Could you check a few things on this model? Use its own coordinates, in mm. Give positions to 0.01 mm unless a question says otherwise; leave off trailing zeros. Loops run counter-clockwise (first coordinate to the right, second up) from the corner with the lowest first, then second, coordinate; pieces in that order, holes last. Notation, with made-up numbers: M -21.5,7 L -1.5,7 A18 cw -1.5,11 Z; hole C 83,32 d9. An arc over 180 degrees is marked long. Write each question's results on one line, items separated by ' | '. Start each with the question number.
from build123d import *

# Parameters (mm, degrees)
F0_R     = 3.175
F1_DEPTH = 31.75
F3_D     = 3.175
F3_DEPTH = 12.7
F3_TIP   = 0.9538662327
F4_SIZE2 = 0.8798818102
F4_SIZE  = 1.524


with BuildPart() as f1:
    # F0 (on Front) → F1 (new body)
    with BuildSketch(Plane.XZ):
        Circle(F0_R)
    extrude(amount=F1_DEPTH)

    # F3
    with Locations(Plane.XZ.offset(31.75)):
        with Locations((0, 0)):
            Hole(F3_D / 2, depth=F3_DEPTH)
            with Locations((0, 0, -(F3_DEPTH + F3_TIP / 2))):  # 118° drill point
                Cone(0, F3_D / 2, F3_TIP, mode=Mode.SUBTRACT)

    # F4
    f4_edges = [f1.edges().sort_by_distance(p)[0] for p in [
        (-3.175, 0, 0),
    ]]
    f4_side = f1.faces().sort_by_distance((-3.175, -15.875, 0))[0]
    chamfer(f4_edges, length=F4_SIZE, length2=F4_SIZE2, reference=f4_side)


solid = f1.part
1) I'm going to push a flat-ended pin straight in: P1, Ø3, axis at x = 0, z = 0, coming from the -Y side. Where does the tip first touch, or does it pass through?
2) Please list where these lines run through material, in increasing order: line 1 (Z direction, x = 0, y = -24) (1 decimal); line 2 (Z direction, x = -0.5, y = -20); line 3 (X direction, y = -26.5, z = 0.75). Write a range as from..to.
3) Thinking about a two-plate mould opening in Z: for faces 1 (the face through (1.4, -31.75, -1.4)), 2 (the face through (-0.69, -16.43, -3.1)), 3 (the face through (0.34, -25.31, -1.55)), which applies, pulls with the +Z half, pulls with the -Z half, needs draft (parallel to the pull), parting line crosses it, or undercut?
4) If we section it at A-A on y = -9.5: Write out the boundary of the cut face in (x, z) (3 decimals), plus the area to 3 significant figures.
Calculated:
1) P1: stops at y = -19
2) line 1: z = -3.2..-1.6, 1.6..3.2 | line 2: z = -3.14..-1.51, 1.51..3.14 | line 3: x = -3.09..-1.4, 1.4..3.09
3) face 1: needs draft | face 2: parting line crosses it | face 3: undercut
4) outline: C 0,0 d6.35 | area: 31.7 mm2
